Read the model definition and answer for the solid it produces. Units are mm, in the model's axes. Round coordinates to 2 decimals unless told otherwise and drop trailing zeros. Use a Markdown table: item, result. Add a question column.
1. Consider L1, parallel to Y at x = 11.6, z = -452; L2, parallel to Y at x = -7.5, z = -435; L3, parallel to Y at x = 0, z = -212.5. Determine where each line is inside the solid, lowest interval first. Write a range as [from, to].
2. Given pin 1 (0.6 mm diameter, centred on y = -14, z = -296, fed in from -X); pin 2 (1.2 mm diameter, centred on y = -2.5, z = -310.5, fed in from -X); pin 3 (4.5 mm diameter, centred on x = 1.5, z = -267, fed in from +Y), each flat-ended and moving along its own axis, determine where each tip first touches the part or whether it passes through.
3. Section A-A, the plane z = -106 is taken. Give the number of separate pieces and of enclosed holes in the cut face, then the cut area to 3 significant figures.
Autodesk Inventor part; units mm, degrees
ref_plane "C1_XY" through (0, 0, 0) normal (0, 0, 1) x (1, 0, 0)
ref_plane "C1_YZ" through (0, 0, 0) normal (1, 0, 0) x (0, 1, 0)
ref_plane "C1_ZX" through (0, 0, 0) normal (0, 1, 0) x (0, 0, 1)
sketch "Sketch_1" plane through (0, 0, 0) normal (0, 0, 1) x (1, 0, 0)
  line L0 (-15, 4) -> (-13, 4)
  line L1 (-13, 4) -> (-13, 8.25)
  line L2 (-13, 8.25) -> (-9.6642, 8.25)
  line L3 (-9.6642, 8.25) -> (-6, 4.5858)
  line L4 (-6, 4.5858) -> (-6, 0.5196)
  line L5 (-6, 0.5196) -> (-5.7, 0)
  line L6 (-5.7, 0) -> (-6, -0.5196)
  line L7 (-6, -0.5196) -> (-6, -4.5858)
  line L8 (-6, -4.5858) -> (-9.6642, -8.25)
  line L9 (-9.6642, -8.25) -> (-13, -8.25)
  line L10 (-13, -8.25) -> (-13, -4)
  line L11 (-13, -4) -> (-15, -4)
  line L12 (-15, -4) -> (-15, -13)
  arc A0 (-15, -13) -> (-13, -15) centre (-13, -13) ccw
  line L13 (-13, -15) -> (-4, -15)
  line L14 (-4, -15) -> (-4, -13)
  line L15 (-4, -13) -> (-8.25, -13)
  line L16 (-8.25, -13) -> (-8.25, -9.6642)
  line L17 (-8.25, -9.6642) -> (-4.5858, -6)
  line L18 (-4.5858, -6) -> (-0.5196, -6)
  line L19 (-0.5196, -6) -> (0, -5.7)
  line L20 (0, -5.7) -> (0.5196, -6)
  line L21 (0.5196, -6) -> (4.5858, -6)
  line L22 (4.5858, -6) -> (8.25, -9.6642)
  line L23 (8.25, -9.6642) -> (8.25, -13)
  line L24 (8.25, -13) -> (4, -13)
  line L25 (4, -13) -> (4, -15)
  line L26 (4, -15) -> (13, -15)
  arc A1 (13, -15) -> (15, -13) centre (13, -13) ccw
  line L27 (15, -13) -> (15, -4)
  line L28 (15, -4) -> (13, -4)
  line L29 (13, -4) -> (13, -8.25)
  line L30 (13, -8.25) -> (9.6642, -8.25)
  line L31 (9.6642, -8.25) -> (6, -4.5858)
  line L32 (6, -4.5858) -> (6, -0.5196)
  line L33 (6, -0.5196) -> (5.7, 0)
  line L34 (5.7, 0) -> (6, 0.5196)
  line L35 (6, 0.5196) -> (6, 4.5858)
  line L36 (6, 4.5858) -> (9.6642, 8.25)
  line L37 (9.6642, 8.25) -> (13, 8.25)
  line L38 (13, 8.25) -> (13, 4)
  line L39 (13, 4) -> (15, 4)
  line L40 (15, 4) -> (15, 13)
  arc A2 (15, 13) -> (13, 15) centre (13, 13) ccw
  line L41 (13, 15) -> (4, 15)
  line L42 (4, 15) -> (4, 13)
  line L43 (4, 13) -> (8.25, 13)
  line L44 (8.25, 13) -> (8.25, 9.6642)
  line L45 (8.25, 9.6642) -> (4.5858, 6)
  line L46 (4.5858, 6) -> (0.5196, 6)
  line L47 (0.5196, 6) -> (0, 5.7)
  line L48 (0, 5.7) -> (-0.5196, 6)
  line L49 (-0.5196, 6) -> (-4.5858, 6)
  line L50 (-4.5858, 6) -> (-8.25, 9.6642)
  line L51 (-8.25, 9.6642) -> (-8.25, 13)
  line L52 (-8.25, 13) -> (-4, 13)
  line L53 (-4, 13) -> (-4, 15)
  line L54 (-4, 15) -> (-13, 15)
  arc A3 (-13, 15) -> (-15, 13) centre (-13, 13) ccw
  line L55 (-15, 13) -> (-15, 4)
extrude "Extrusion1" add sketch "Sketch_1" against normal blind 600
sketch "Sketch2" plane through (0, 0, -600) normal (0, 0, -1) x (-1, 0, 0)
  point P0 (0, 0)
hole "Hole1" at (0, 0, -600) direction (0, 0, 1) diameter 6.8 depth 600
sketch "Sketch3" plane through (0, 0, -600) normal (0, 0, -1) x (-1, 0, 0)
  point P0 (-11.6, 11.6)
hole "Hole2" at (11.6, 11.6, -600) direction (0, 0, 1) diameter 4.2 depth 600
pattern_linear "Rectangular Pattern1" count 2 spacing 23.2 along (-1, 0, 0) count 2 spacing 23.2 along (0, -1, 0) of "Hole2"
ref_plane "C1_XY" through (0, 0, 0) normal (0, 0, 1) x (1, 0, 0)
ref_plane "C1_YZ" through (0, 0, 0) normal (1, 0, 0) x (0, 1, 0)
ref_plane "C1_ZX" through (0, 0, 0) normal (0, 1, 0) x (0, 0, 1)
ref_plane "to_frame_cap1_XY" through (0, 0, 0) normal (0, 0, 1) x (1, 0, 0)
ref_plane "to_frame_cap1_YZ" through (0, 0, 0) normal (1, 0, 0) x (0, 1, 0)
ref_plane "to_frame_cap1_ZX" through (0, 0, 0) normal (0, 1, 0) x (0, 0, 1)
ref_plane "to_frame_cap2_XY" through (0, 0, -600) normal (0, 0, -1) x (1, 0, 0)
ref_plane "to_frame_cap2_YZ" through (0, 0, -600) normal (1, 0, 0) x (0, -1, 0)
ref_plane "to_frame_cap2_ZX" through (0, 0, -600) normal (0, -1, 0) x (0, 0, -1)
properties part number "HFS6-3030-600"
Verdict:
| question | item | result |
|---|---|---|
| 1 | L1 | y = [-15, -13.7], [-9.5, -8.25], [8.25, 9.5], [13.7, 15] |
| 1 | L2 | y = [-15, -13], [-8.91, -6.09], [6.09, 8.91], [13, 15] |
| 1 | L3 | y = [-5.7, -3.4], [3.4, 5.7] |
| 2 | pin 1 | stops at x = -14.87 |
| 2 | pin 2 | stops at x = -6 |
| 2 | pin 3 | stops at y = 6 |
| 3 | separate pieces | 1 |
| 3 | enclosed holes | 5 |
| 3 | area | 332 mm2 |
